Part print with two shaded views. Sizes in mm from the minimum x, y, z corner. Round coordinates to 2 decimals unless told otherwise and drop trailing zeros. Write each loop counter-clockwise with the first axis right and the second up, starting at its lowest first coordinate (ties: lowest second). Pieces come first, ordered by that corner, then holes. Notation, with made-up numbers: (-32.5, 19) -> (-25.5, 19) arc R8 cw to (-25.5, 32) -> close; hole circle Ø8 at (35, -38). An arc over 180 degrees is marked (long way). Answer in a Markdown table with one row per item.
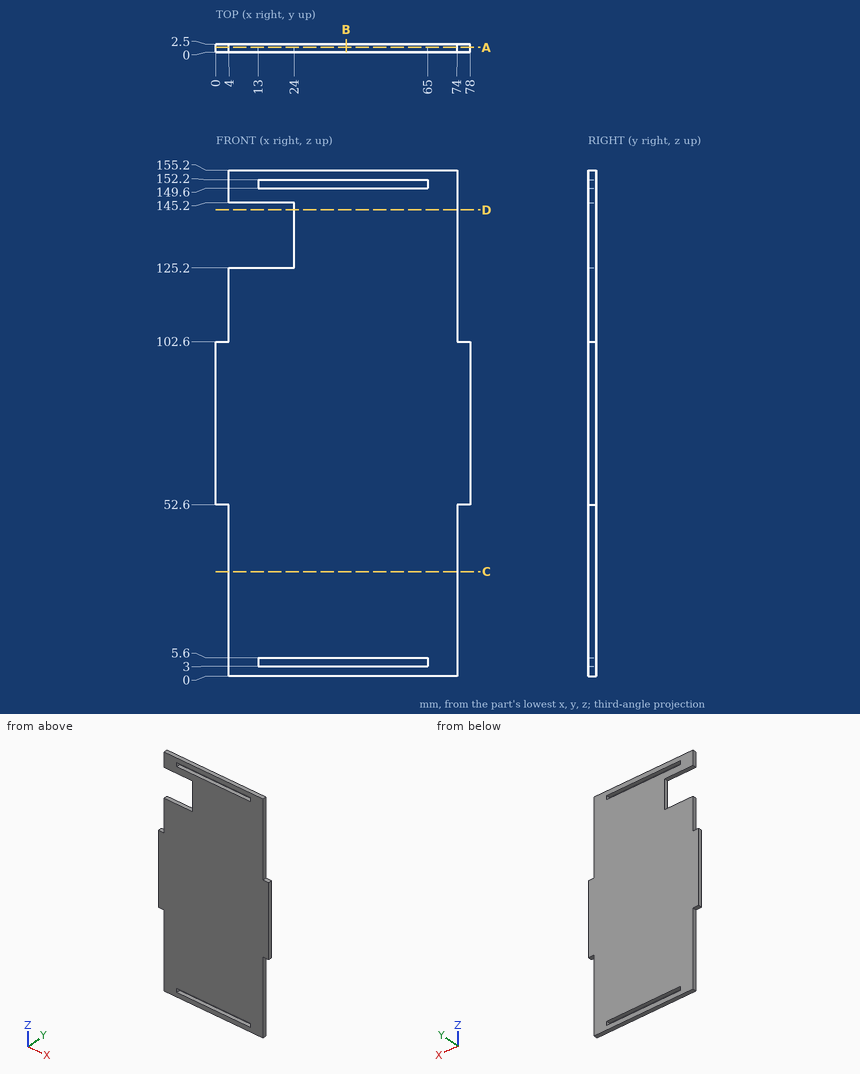
Q1. Saw through at B-B on x = 40. Write the cut outline in (y, z), plus the area to 3 significant figures.
A:
| item | result |
|---|---|
| outline | (0, 0) -> (2.5, 0) -> (2.5, 3) -> (0, 3) -> close; (0, 5.6) -> (2.5, 5.6) -> (2.5, 149.6) -> (0, 149.6) -> close; (0, 152.2) -> (2.5, 152.2) -> (2.5, 155.2) -> (0, 155.2) -> close |
| area | 375 mm² |
Q2. Saw through at D-D on z = 143. Write the cut outline in (x, y), plus the area to 3 significant figures.
A:
| item | result |
|---|---|
| outline | (24, 0) -> (74, 0) -> (74, 2.5) -> (24, 2.5) -> close |
| area | 125 mm² |
Q3. Drop flat-ended pins along their axis: P1, Ø0.8, axis at y = 0.5, z = 148, coming from the -X side; P2, Ø1.2, axis at x = 3, y = 1.5, coming from the +Z side; P3, Ø0.8, axis at x = 3, y = 1, coming from the -Z side. Give the stop position or say it passes through.
A:
| item | result |
|---|---|
| P1 | x = 4 |
| P2 | z = 102.6 |
| P3 | z = 52.6 |
Q4. Saw through at A-A on y = 1.45. Write the cut outline in (x, z), plus the area to 3 significant figures.
A:
| item | result |
|---|---|
| outline | (0, 52.6) -> (4, 52.6) -> (4, 0) -> (74, 0) -> (74, 52.6) -> (78, 52.6) -> (78, 102.6) -> (74, 102.6) -> (74, 155.2) -> (4, 155.2) -> (4, 145.2) -> (24, 145.2) -> (24, 125.2) -> (4, 125.2) -> (4, 102.6) -> (0, 102.6) -> close; hole (13, 3) -> (65, 3) -> (65, 5.6) -> (13, 5.6) -> close; hole (13, 149.6) -> (65, 149.6) -> (65, 152.2) -> (13, 152.2) -> close |
| area | 10,600 mm² |
Q5. Wall check: line 1 (Z direction, x = 29, y = 0.3); line 2 (Z direction, x = 16.5, y = 2.2); line 3 (Z direction, x = 10.5, y = 1.2). Give the ranges that are in metal, low to high. Write a range as [from, to].
A:
| item | result |
|---|---|
| line 1 | [0, 3], [5.6, 149.6], [152.2, 155.2] |
| line 2 | [0, 3], [5.6, 125.2], [145.2, 149.6], [152.2, 155.2] |
| line 3 | [0, 125.2], [145.2, 155.2] |
Q6. Saw through at C-C on z = 32. Write the cut outline in (x, y), plus the area to 3 significant figures.
A:
| item | result |
|---|---|
| outline | (4, 0) -> (74, 0) -> (74, 2.5) -> (4, 2.5) -> close |
| area | 175 mm² |
